Work out the finished part from the listing and answer in its coordinate system (mm). Face numbers are marked on the shaded views. A direction names the side the tool comes from. Coordinates: 2 decimals unless noted, no trailing zeros. Order: outer loops, then holes, each group sorted by start corner. A loop starts at its lowest first (then second) coordinate and runs counter-clockwise, first axis right, second up. Notation, with made-up numbers: (48, 13.5) - (60, 13.5) arc R22 ccw to (60, 49.5) - close; hole circle Ø7 at (42, 50.25). An arc over 180 degrees is marked (long way). Answer as a JSON object with one key per item and string values. Group by question number.
1) A tool of negligible diameter and unlimited length cuts with its end or side. For the marked faces 4 and 5, from which of +Z, -Z, +X, -X, +Y, -Y can it reach the whole face along a straight path? Write none if from no direction.
2) Section B-B (y = 37.5) is taken. Give the vertices of the cut face in (x, z).
3) The mould has two halves that part along X. Classify the marked faces 1, 2 and 3: released by +X, released by -X, zero draft, split by the parting line, or undercut.
4) Each of these flat-tipped pins is pushed along its axis until it touches: P1, Ø12, axis at x = 92, z = 22, coming from the -Y side; P2, Ø1.2, axis at x = -73.5, y = 4.5, coming from the -Z side; P3, Ø8, axis at y = 46, z = 26.5, coming from the +X side. Where does it stop, or does it pass through?
5) Section C-C (z = 49) is taken. Give the vertices of the cut face in (x, y), plus the area to 3 significant figures.
6) Section A-A (z = 65) is taken. Give the vertices of the cut face in (x, y), plus the area to 3 significant figures.
7) Section D-D (x = -46) is taken. Give the vertices of the cut face in (y, z), plus the area to 3 significant figures.
8) Find the intervals of material crossed by line 1 along X through (y, z) = (80, 39.5); line 2 along X through (y, z) = (46.5, 48); line 3 along Y through (x, z) = (-45, 43), in increasing order.
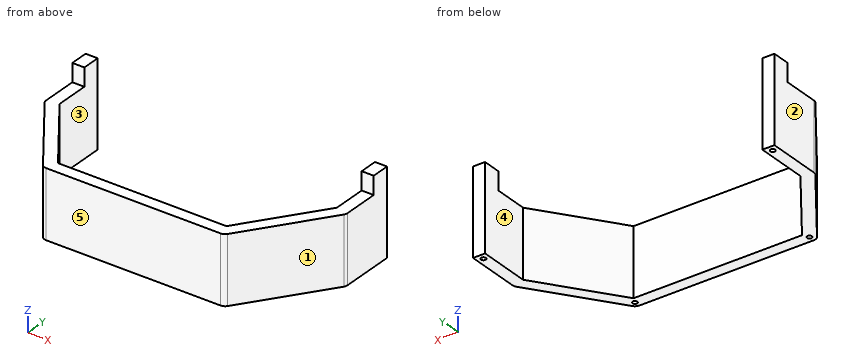
from build123d import *

# Parameters (mm, degrees)
BOSS_EXTRU_1_DEPTH      = 71
ESQUISSE3_W             = 324.913222196
ESQUISSE3_H             = 116.889512864
ENL_V_MAT_EXTRU_2_DEPTH = 15
CONG_1_R                = 5
ESQUISSE4_R             = 2
ENL_V_MAT_EXTRU_3_DEPTH = 8


with BuildPart() as part:
    # Esquisse1 → Boss.-Extru.1 (new body)
    with BuildSketch(Plane.XY):
        Polygon((-124.99814732, 116.197326124), (-114.99814732, 116.197326124), (-114.99814732, 73.201979643), (-69.853824471, 10), (69.854159245, 10), (115.001852666, 73.199624684), (115.001852666, 116.194679298), (125.001852666, 116.194679298), (125.001852666, 69.994679298), (75, 0), (-75, 0), (-124.99814732, 69.997326124), align=None)
    extrude(amount=BOSS_EXTRU_1_DEPTH)

    # Esquisse3 → Enlèv. mat.-Extru.2 (cut)
    with BuildSketch(Plane.XY.offset(71)):
        with Locations((-2.475787976, 42.749922866)):
            Rectangle(ESQUISSE3_W, ESQUISSE3_H)
    extrude(amount=-ENL_V_MAT_EXTRU_2_DEPTH, mode=Mode.SUBTRACT)

    # Congé1
    cong_1_edges = [part.edges().sort_by_distance(p)[0] for p in [
        (125.001852666, 69.994679298, 28),
        (75, 0, 28),
        (-75, 0, 28),
        (-124.99814732, 69.997326124, 28),
    ]]
    fillet(cong_1_edges, radius=CONG_1_R)

    # Esquisse4 → Enlèv. mat.-Extru.3 (cut)
    with BuildSketch(Plane(origin=(0, 0, 0), x_dir=(-1, 0, 0), z_dir=(0, 0, -1))):
        with Locations((-72.427079623, 5)):
            Circle(ESQUISSE4_R)
        with Locations((72.426912235, 5)):
            Circle(ESQUISSE4_R)
        with Locations((-120.001852666, 111.194679298)):
            Circle(ESQUISSE4_R)
        with Locations((119.99814732, 111.197326124)):
            Circle(ESQUISSE4_R)
    extrude(amount=-ENL_V_MAT_EXTRU_3_DEPTH, mode=Mode.SUBTRACT)


solid = part.part
Report:
{
 "1": {"face 4": "+Z, -Z, +Y", "face 5": "+Z, -Z, +X, -X, -Y"},
 "2": {"outline": "(-101.79, 0) - (-89.5, 0) - (-89.5, 56) - (-101.79, 56) - close; (89.5, 0) - (101.79, 0) - (101.79, 56) - (89.5, 56) - close"},
 "3": {"face 1": "released by +X", "face 2": "released by -X", "face 3": "undercut"},
 "4": {"P1": "stops at y = 15.4", "P2": "stops at z = 8", "P3": "stops at x = 110.72"},
 "5": {"outline": "(-125, 71.6) arc R5 ccw to (-124.07, 68.69) - (-76.5, 2.09) arc R5 ccw to (-72.43, 0) - (72.43, 0) arc R5 ccw to (76.5, 2.09) - (124.07, 68.69) arc R5 ccw to (125, 71.6) - (125, 116.19) - (115, 116.19) - (115, 73.2) - (69.85, 10) - (-69.85, 10) - (-115, 73.2) - (-115, 116.2) - (-125, 116.2) - close", "area": "3,970 mm²"},
 "6": {"outline": "(-125, 101.19) - (-115, 101.19) - (-115, 116.2) - (-125, 116.2) - close; (115, 101.19) - (125, 101.19) - (125, 116.19) - (115, 116.19) - close", "area": "300 mm²"},
 "7": {"outline": "(0, 0) - (10, 0) - (10, 56) - (0, 56) - close", "area": "560 mm²"},
 "8": {"line 1": "x = -125 to -115, 115 to 125", "line 2": "x = -108.21 to -95.93, 95.93 to 108.22", "line 3": "y = 0 to 10"}
}
